Here's how the part is built. I have some questions about the finished solid (model axes, mm). A direction names the side the tool comes from. Give positions to 0.01 mm unless a question says otherwise; leave off trailing zeros. Write each loop counter-clockwise with the first axis right and the second up, starting at its lowest first coordinate (ties: lowest second). Pieces come first, ordered by that corner, then holes. Notation, with made-up numbers: M 72.25,43 L 85.25,43 A6 cw 85.25,53 Z; hole C 1,-35.5 d9. An arc over 180 degrees is marked long. Answer as CSV lines item,"result". Start each with the question number.
Q1. Suppose I cut it at C-C (z = 1). Write out the boundary of the cut face in (x, y) (3 decimals).
Q2. Suppose I cut it at A-A (x = 0). Write out the boundary of the cut face in (y, z) (3 decimals), then the cut area to 3 significant figures.
Q3. If I drill on line 1 along Y through (x, z) = (0, 11.2) (3 decimals); line 2 along Z through (x, y) = (-6.5, 0.75); line 3 along Z through (x, y) = (12, 4.25), over which ranges is the centre line in solid material (lowest first)?
Q4. Thinking about a two-plate mould opening in Y: for faces 1 (the flat face through (0, -13.97, 3)), 2 (the cylindrical face through (-9.45, -7.24, 8.64)), 3 (the cylindrical face through (-12.154, 12.053, 2.936)), 4 (the flat face through (13.97, 0, 3)), which applies, +Y half, -Y half, draft (parallel to the pull), parting line (faces both ways), or undercut?
Q5. For pin 1 (1.5 mm diameter, centred on x = 8.5, z = -27.5, fed in from -Y); pin 2 (5 mm diameter, centred on y = -3.5, z = -5, fed in from -X); pin 3 (2 mm diameter, centred on x = -10.945, y = 10.945, fed in from +Z); pin 4 (6 mm diameter, centred on x = 0, z = -27.5, fed in from -Y), each with a flat end and sliding along its axis, tell me the tip position at first contact or that it passes through.
Q6. Suppose I cut it at D-D (z = -42). Write out the boundary of the cut face in (x, y), then the cut area to 3 significant figures.
Q7. On a 3-axis mill with a long thin cutter (end or side, diameter ignored), from which of +Z, -Z, +X, -X, +Y, -Y can I reach the whole of each face in a straight line? I mean faces 5 (the flat face through (12.2, 0.2, 5.79)), 6 (the flat face through (3, 12.5, 0)), 7 (the cylindrical face through (12.51, -10.45, 2.94)). Say none if no direction works.
```python
from build123d import *

# Parameters (mm, degrees)
SKETCH2_W           = 27.94
SKETCH2_H           = 27.94
BOSS_EXTRUDE1_DEPTH = 5.79
SKETCH3_R           = 11.905
BOSS_EXTRUDE2_DEPTH = 5.79
SKETCH4_R           = 4.765
BOSS_EXTRUDE3_DEPTH = 9.12
SKETCH5_R           = 12.7
BOSS_EXTRUDE4_DEPTH = 65.25
CUT_EXTRUDE1_START  = -0.75
SKETCH6_R           = 10.648931608
SKETCH6_R_2         = 4.765
CUT_EXTRUDE1_DEPTH  = 0.75
SKETCH7_R           = 7.420951144
BOSS_EXTRUDE5_DEPTH = 0.5
SKETCH8_R           = 6.651278865
BOSS_EXTRUDE6_DEPTH = 0.5
SKETCH9_R           = 1.64
CUT_EXTRUDE2_DEPTH  = 10.5


with BuildPart() as part:
    # Sketch2 → Boss-Extrude1 (new body)
    with BuildSketch(Plane.XY):
        Rectangle(SKETCH2_W, SKETCH2_H)
    extrude(amount=BOSS_EXTRUDE1_DEPTH)

    # Sketch3 → Boss-Extrude2 (add)
    with BuildSketch(Plane.XY.offset(5.79)):
        Circle(SKETCH3_R)
    extrude(amount=BOSS_EXTRUDE2_DEPTH)

    # Sketch4 → Boss-Extrude3 (add)
    with BuildSketch(Plane.XY.offset(11.58)):
        Circle(SKETCH4_R)
    extrude(amount=BOSS_EXTRUDE3_DEPTH)

    # Sketch5 → Boss-Extrude4 (add)
    with BuildSketch(Plane(origin=(0, 0, 0), x_dir=(-1, 0, 0), z_dir=(0, 0, -1))):
        Circle(SKETCH5_R)
    extrude(amount=BOSS_EXTRUDE4_DEPTH)

    # Sketch6 → Cut-Extrude1 (cut)
    with BuildSketch(Plane.XY.offset(11.58).offset(CUT_EXTRUDE1_START)):
        Circle(SKETCH6_R)
        Circle(SKETCH6_R_2, mode=Mode.SUBTRACT)
    extrude(amount=CUT_EXTRUDE1_DEPTH, mode=Mode.SUBTRACT)

    # Sketch7 → Boss-Extrude5 (add)
    with BuildSketch(Plane.XY.offset(10.83)):
        Circle(SKETCH7_R)
    extrude(amount=BOSS_EXTRUDE5_DEPTH)

    # Sketch8 → Boss-Extrude6 (add)
    with BuildSketch(Plane.XY.offset(11.33)):
        Circle(SKETCH8_R)
    extrude(amount=BOSS_EXTRUDE6_DEPTH)

    # Sketch9 → Cut-Extrude2 (cut)
    with BuildSketch(Plane.XY.offset(5.79)):
        with Locations((-10.945, 10.945)):
            Circle(SKETCH9_R)
        with Locations((10.945, 10.945)):
            Circle(SKETCH9_R)
        with Locations((10.945, -10.945)):
            Circle(SKETCH9_R)
        with Locations((-10.945, -10.945)):
            Circle(SKETCH9_R)
    extrude(amount=-CUT_EXTRUDE2_DEPTH, mode=Mode.SUBTRACT)


solid = part.part
```
Resolved:
1,outline,"M -13.97,-13.97 L 13.97,-13.97 L 13.97,13.97 L -13.97,13.97 Z; hole C -10.945,-10.945 d3.28; hole C -10.945,10.945 d3.28; hole C 10.945,-10.945 d3.28; hole C 10.945,10.945 d3.28"
2,outline,"M -13.97,0 L -12.7,0 L -12.7,-65.25 L 12.7,-65.25 L 12.7,0 L 13.97,0 L 13.97,5.79 L 11.905,5.79 L 11.905,11.58 L 10.649,11.58 L 10.649,10.83 L 7.421,10.83 L 7.421,11.33 L 6.651,11.33 L 6.651,11.83 L 4.765,11.83 L 4.765,20.7 L -4.765,20.7 L -4.765,11.83 L -6.651,11.83 L -6.651,11.33 L -7.421,11.33 L -7.421,10.83 L -10.649,10.83 L -10.649,11.58 L -11.905,11.58 L -11.905,5.79 L -13.97,5.79 Z"
2,area,"2,040 mm^2"
3,line 1,"-11.905 to -10.649, -7.421 to 7.421, 10.649 to 11.905"
3,line 2,"-65.25 to 11.83"
3,line 3,"0 to 5.79"
4,face 1,"-Y half"
4,face 2,"parting line"
4,face 3,"undercut"
4,face 4,"draft"
5,pin 1,"y = -10.06"
5,pin 2,"x = -12.66"
5,pin 3,"through"
5,pin 4,"y = -12.7"
6,outline,"C 0,0 d25.4"
6,area,"507 mm^2"
7,face 5,"+Z"
7,face 6,"-Z"
7,face 7,"+Z, -Z"
